```python
from build123d import *

# Parameters (mm, degrees)
SKETCH_1_R          = 7.5
EXTRUDE_1_DEPTH     = 5
EXTRUDE_2_DEPTH     = 5
SKETCH_3_R          = 7.5
EXTRUDE_3_DEPTH     = 1
EXTRUDE_4_DEPTH     = 4.5
EXTRUDE_5_DEPTH     = 10
SKETCH_6_R          = 9
EXTRUDE_6_DEPTH     = 0.1
DOME_1_FACE_RADIUS  = 9
DOME_1_HEIGHT       = 7
SKETCH_7_R          = 5.5
CUT_EXTRUDE_1_DEPTH = 24.5
SKETCH_8_R          = 4
CUT_EXTRUDE_2_DEPTH = 20
SKETCH_9_W          = 14.275225046
SKETCH_9_H          = 13.315546052
CUT_EXTRUDE_3_DEPTH = 20


with BuildPart() as part:
    # Эскиз1 → Вытянуть1 (new body)
    with BuildSketch(Plane.XY):
        Circle(SKETCH_1_R)
    extrude(amount=-EXTRUDE_1_DEPTH)

    # Эскиз2 → Вытянуть2 (add)
    with BuildSketch(Plane(origin=(0, 0, -5), x_dir=(-1, 0, 0), z_dir=(0, 0, -1))):
        Polygon((0, 12.701705922), (-11, 6.350852961), (-11, -6.350852961), (0, -12.701705922), (11, -6.350852961), (11, 6.350852961), align=None)
    extrude(amount=EXTRUDE_2_DEPTH)

    # Эскиз3 → Вытянуть3 (add)
    with BuildSketch(Plane(origin=(0, 0, -10), x_dir=(-1, 0, 0), z_dir=(0, 0, -1))):
        with Locations(Location((0, 0, 0), (0, 0, 180))):
            Circle(SKETCH_3_R)
    extrude(amount=EXTRUDE_3_DEPTH)

    # Эскиз4 → Вытянуть4 (add)
    with BuildSketch(Plane(origin=(0, 0, -11), x_dir=(-1, 0, 0), z_dir=(0, 0, -1))):
        Polygon((0, 10.392304845), (-9, 5.196152423), (-9, -5.196152423), (0, -10.392304845), (9, -5.196152423), (9, 5.196152423), align=None)
    extrude(amount=EXTRUDE_4_DEPTH)

    # Эскиз5 → Вытянуть5 (add)
    with BuildSketch(Plane(origin=(0, 0, -15.5), x_dir=(-1, 0, 0), z_dir=(0, 0, -1))):
        Polygon((0, 10.969655115), (-9.5, 5.484827557), (-9.5, -5.484827557), (0, -10.969655115), (9.5, -5.484827557), (9.5, 5.484827557), align=None)
    extrude(amount=EXTRUDE_5_DEPTH)

    # Эскиз6 → Вытянуть6 (add)
    with BuildSketch(Plane(origin=(0, 0, -25.5), x_dir=(-1, 0, 0), z_dir=(0, 0, -1))):
        with Locations(Location((0, 0, 0), (0, 0, 180))):
            Circle(SKETCH_6_R)
    extrude(amount=EXTRUDE_6_DEPTH)

    # Купол1: a dome of height H over a round flat face of radius A is a cap of a sphere of radius (A * A + H * H) / (2 * H)
    dome_1_r = (DOME_1_FACE_RADIUS * DOME_1_FACE_RADIUS + DOME_1_HEIGHT * DOME_1_HEIGHT) / (2 * DOME_1_HEIGHT)
    dome_1_base = Plane((0, 0, -25.6), z_dir=(0, 0, -1))
    with Locations(dome_1_base.offset(DOME_1_HEIGHT - dome_1_r)):
        dome_1_ball = Sphere(dome_1_r, mode=Mode.PRIVATE)
    add(split(dome_1_ball, bisect_by=dome_1_base, keep=Keep.TOP, mode=Mode.PRIVATE))

    # Эскиз7 → Вырез-Вытянуть1 (cut)
    with BuildSketch(Plane.XY):
        Circle(SKETCH_7_R)
    extrude(amount=-CUT_EXTRUDE_1_DEPTH, mode=Mode.SUBTRACT)

    # Эскиз8 → Вырез-Вытянуть2 (cut)
    with BuildSketch(Plane.XY.offset(-24.5)):
        Circle(SKETCH_8_R)
    extrude(amount=-CUT_EXTRUDE_2_DEPTH, mode=Mode.SUBTRACT)

    # Эскиз9 → Вырез-Вытянуть3 (cut)
    with BuildSketch(Plane.XY.offset(-31)):
        with Locations((-0.20992978, 0.329889654)):
            Rectangle(SKETCH_9_W, SKETCH_9_H)
    extrude(amount=-CUT_EXTRUDE_3_DEPTH, mode=Mode.SUBTRACT)


solid = part.part
```
Verification items for the finished model (mm, model axes). A direction names the side the tool comes from. Give positions to 0.01 mm unless a question says otherwise; leave off trailing zeros. Order: outer loops, then holes, each group sorted by start corner. A loop starts at its lowest first (then second) coordinate and runs counter-clockwise, first axis right, second up. Notation, with made-up numbers: M 16.25,-19 L 27.25,-19 A22 ccw 27.25,19 Z; hole C 20,65 d6. An arc over 180 degrees is marked long. Return JSON: item names as keys, results as strings. Group by question number.
1) Mould release check, pull along X, two halves, no side actions. Record for faces 5 (the face through (-4.56, 7.76, -13.22)), 6 (the face through (5.423, 9.571, -7.465)), 7 (the face through (-4, -2, -24.5)): pulls with the +X half, pulls with the -X half, needs draft (parallel to the pull), parting line crosses it, or undercut.
2) Scan lines: line 1 (Z direction, x = 2.5, y = 9); line 2 (Y direction, x = 0, z = -8); line 3 (Z direction, x = 7.75, y = 5.5). Record each from-to range of solid material in increasing order.
3) Go/stop test with flat-tipped pins: pin 1 Ø12 at (x, y) = (-1, 7) entering from -Z; pin 2 Ø2 at (x, z) = (-3, -5.5) entering from +Y; pin 3 Ø2 at (y, z) = (2.5, -12) entering from +X; pin 4 Ø8 at (y, z) = (0.5, -20.5) entering from -X. Record where each tip stops, or that it passes through.
4) Access from +Z, -Z, +X, -X, +Y, -Y to the whole of each face (thin tool, end or side, straight path). Record for faces 1 (the face through (-7.493, 0.33, -2.465)), 2 (the face through (-7.2, -2.6, -10)), 3 (the face through (9.5, 0, -20)), 4 (the face through (-4.44, -7.83, -13.22)).
5) Section check D-D on z = -22. Record the cut outline in (x, y).
6) Section check B-B on z = -12. Record the cut outline in (x, y).
Answer block:
{
 "1": {"face 5": "pulls with the -X half", "face 6": "pulls with the +X half", "face 7": "undercut"},
 "2": {"line 1": "z = -25.5 to -15.5, -10 to -5", "line 2": "y = -12.7 to -5.5, 5.5 to 12.7", "line 3": "z = -25.5 to -11, -10 to -5"},
 "3": {"pin 1": "stops at z = -31", "pin 2": "stops at y = 11.55", "pin 3": "stops at x = 9", "pin 4": "stops at x = -9.5"},
 "4": {"face 1": "+Z", "face 2": "none", "face 3": "-Z, +X, +Y, -Y", "face 4": "-X, -Y"},
 "5": {"outline": "M -9.5,-5.48 L 0,-10.97 L 9.5,-5.48 L 9.5,5.48 L 0,10.97 L -9.5,5.48 Z; hole C 0,0 d11"},
 "6": {"outline": "M -9,-5.2 L 0,-10.39 L 9,-5.2 L 9,5.2 L 0,10.39 L -9,5.2 Z; hole C 0,0 d11"}
}
